For this review, take the finished solid that the model builds, in its own axes (mm). Give positions to 0.01 mm unless a question says otherwise; leave off trailing zeros. Loops run counter-clockwise (first coordinate to the right, second up) from the corner with the lowest first, then second, coordinate; pieces in that order, holes last. Notation, with made-up numbers: (55, 29.5) - (108, 29.5) arc R22 cw to (108, 37.5) - close; hole circle Ø5 at (27, -15.75). An arc over 180 degrees is marked (long way). Use CSV: the item, a comma, the result in double quotes. Start each with the question number.
1. Take a section at C-C on y = 0.6. Give the boundary of the cut face in (x, z), plus the area to 3 significant figures.
2. Wall thickness on line 1 (X direction, y = 2.1, z = 0); line 2 (Z direction, x = 0, y = 2.3): over which ranges is each line inside the solid? List them lowest first.
3. For pin 1 (1 mm diameter, centred on x = -8, y = 0.5, fed in from +Z); pin 2 (3 mm diameter, centred on x = 38.5, z = -0.5, fed in from -Y); pin 3 (1 mm diameter, centred on x = -6.5, y = 3, fed in from +Z), all flat-tipped, find the tip position at first contact; note any pin that passes through.
4. Take a section at A-A on x = 0. Give the boundary of the cut face in (y, z).
5. Take a section at B-B on z = 0. Give the boundary of the cut face in (x, y).
6. Take a section at D-D on x = 21.5. Give the boundary of the cut face in (y, z).
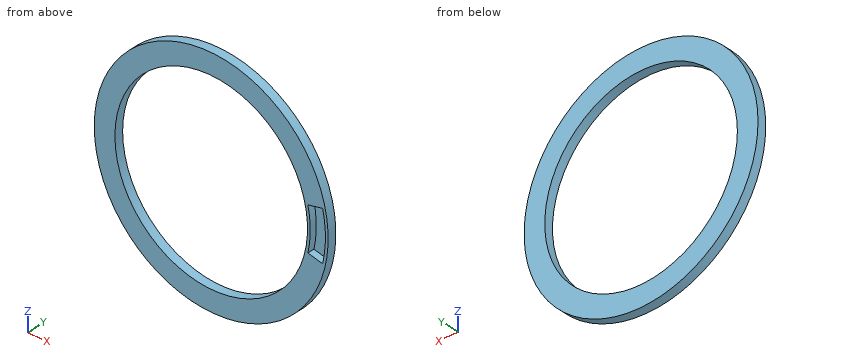
Autodesk Inventor part; units mm, degrees
ref_plane "YZ Plane" through (0, 0, 0) normal (1, 0, 0) x (0, 1, 0)
ref_plane "XZ Plane" through (0, 0, 0) normal (0, 1, 0) x (-1, 0, 0)
ref_plane "XY Plane" through (0, 0, 0) normal (0, 0, 1) x (1, 0, 0)
sketch "Sketch1" plane through (0, 0, 0) normal (0, 1, 0) x (-1, 0, 0)
  circle A0 centre (0, 0) radius 42.5
  circle A1 centre (0, 0) radius 35
  line L0 (0, 0) -> (-41.3068, 10)
  line L1 (0, 0) -> (-41.3068, -10)
  line L2 (0, 0) -> (-42.5, 0)
  line L3 (-28.5133, 6.9028) -> (-28.5133, -6.9028)
  arc A2 (-34.9893, 8.4706) -> (-34.9893, -8.4706) centre (0, 0) ccw
  arc A3 (-40.3349, 9.7647) -> (-40.3349, -9.7647) centre (0, 0) ccw
  line L4 (0, 0) -> (-41.475, 9.2776)
  line L5 (0, 0) -> (-41.475, -9.2776)
  point P0 (-28.5133, 0)
  point P1 (-40.4991, -9.0593)
  point P2 (-35.1318, -7.8587)
  point P3 (-35.1318, 7.8587)
  point P4 (-40.4991, 9.0593)
  dimension "d0" = 85
  dimension "d1" = 70
  dimension "d2" = 20
  dimension "d4" = 1
  dimension "d5" = 1
  dimension "d6" = 1
  dimension "d7" = 1
extrude "Extrusion1" add sketch "Sketch1" along normal blind 3.2 contours A0 L1 A1 L0 | L0 A3 L4 A0 | A0 L5 A3 L1 | L4 A3 L2 A0 | L0 A2 L4 A3 | A0 L2 A3 L5 | A3 L5 A2 L1 | L4 A2 L2 A3 | L0 A1 L4 A2 | A3 L2 A2 L5 | A2 L5 A1 L1 | L4 A1 L2 A2 | A2 L2 A1 L5
extrude "Extrusion2" cut sketch "Sketch1" along normal blind 2.5 contours L4 A2 L2 A3 | A3 L2 A2 L5
properties part number "NeoPixel-24"
Check result:
1,outline,"circle Ø85 at (0, 0); hole circle Ø70 at (0, 0); hole (35.13, -7.86) - (40.5, -9.06) arc R41.5 ccw to (40.5, 9.06) - (35.13, 7.86) arc R36 cw to start"
1,area,"1,730 mm²"
2,line 1,"x = -42.5 to -35, 35 to 36, 41.5 to 42.5"
2,line 2,"z = -42.5 to -35, 35 to 42.5"
3,pin 1,"stops at z = 41.83"
3,pin 2,"stops at y = 2.5"
3,pin 3,"stops at z = 42.07"
4,outline,"(0, -42.5) - (3.2, -42.5) - (3.2, -35) - (0, -35) - close; (0, 35) - (3.2, 35) - (3.2, 42.5) - (0, 42.5) - close"
5,outline,"(-42.5, 0) - (-35, 0) - (-35, 3.2) - (-42.5, 3.2) - close; (35, 0) - (36, 0) - (36, 2.5) - (41.5, 2.5) - (41.5, 0) - (42.5, 0) - (42.5, 3.2) - (35, 3.2) - close"
6,outline,"(0, -36.66) - (3.2, -36.66) - (3.2, -27.62) - (0, -27.62) - close; (0, 27.62) - (3.2, 27.62) - (3.2, 36.66) - (0, 36.66) - close"
